```python
from build123d import *

# Parameters (mm, degrees)
F1_DEPTH = 15
F2_R     = 4
F3_DEPTH = 5


with BuildPart() as f1:
    # F0 (on Front) → F1 (new body, symmetric)
    with BuildSketch(Plane.XZ):
        with BuildLine():
            Line((0, 50), (-50, 50))
            Line((-50, 50), (-50, -50))
            Line((-50, -50), (0, -50))
            Line((0, -50), (0, -30))
            Line((0, -30), (-10, -30))
            ThreePointArc((-10, -30), (-18, -22.5), (-10, -15))
            Line((-10, -15), (0, -15))
            Line((0, -15), (0, 50))
        make_face()
    extrude(amount=F1_DEPTH, both=True)

    # F2 (on face) → F3 (cut)
    with BuildSketch(Plane.XZ.offset(15)):
        with Locations((-25, 25)):
            Circle(F2_R)
    extrude(amount=-F3_DEPTH, mode=Mode.SUBTRACT)


solid = f1.part
```
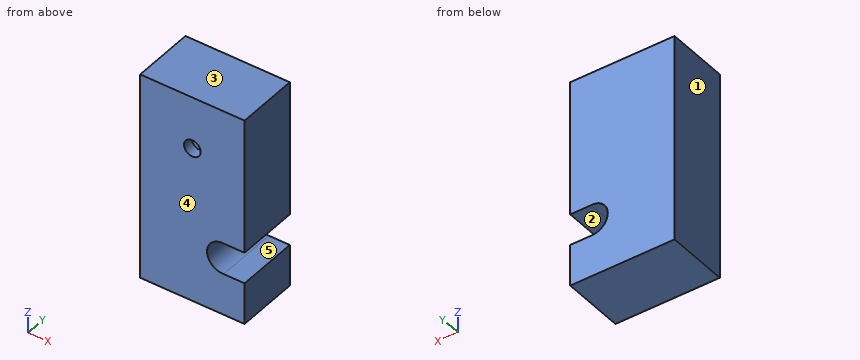
Source: CAD feature listing. Evaluate the final solid. Frame: model axes, mm. Face numbers are marked on the shaded views. A direction names the side the tool comes from. Give positions to 0.01 mm unless a question says otherwise; leave off trailing zeros. Loops run counter-clockwise (first coordinate to the right, second up) from the corner with the lowest first, then second, coordinate; pieces in that order, holes last. Notation, with made-up numbers: (24, 52.5) -> (38, 52.5) arc R12 cw to (38, 57.5) -> close; hole circle Ø9 at (24, 13.5). An arc over 180 degrees is marked (long way). Use a Markdown table: item, result. Add a question column.
(1) Section query C-C (y = -1.25). Output: boundary loops of the cut face in (x, z), then the cut area to 3 significant figures.
(2) Access query for the marked faces 4 and 5. Directions: +Z, -Z, +X, -X, +Y, -Y. A direction counts if a zero-diameter tool reaches every point of the face in a straight line with its end or side. Return the directions, or none.
(3) First-contact query: pin 1 Ø5 at (x, z) = (-25, 25) entering from -Y; pin 2 Ø9 at (x, z) = (-24, 25.5) entering from -Y. Flat tips, straight axial feed; report the tip coordinate or a pass-through.
(4) Pull-direction query (Z, two-part tool) for the marked faces 1, 2 and 3; classes: +Z half, -Z half, draft (parallel to the pull), parting line (faces both ways), or undercut.
(5) Section query B-B (y = -11.75). Output: boundary loops of the cut face in (x, z), then the cut area to 3 significant figures.
(6) Section query D-D (z = 25). Output: boundary loops of the cut face in (x, y), then the cut area to 3 significant figures.
(7) Ray query, line 1 (Z direction, x = -25, y = -12.35); line 2 (Z direction, x = -3, y = -9.5); line 3 (X direction, y = -1, z = -28.5). Return the intervals inside material, ascending.
(8) Section query A-A (x = -5.5). Output: boundary loops of the cut face in (y, z), then the cut area to 3 significant figures.
Checked values:
| question | item | result |
|---|---|---|
| 1 | outline | (-50, -50) -> (0, -50) -> (0, -30) -> (-10, -30) arc R7.52 cw (long way) to (-10, -15) -> (0, -15) -> (0, 50) -> (-50, 50) -> close |
| 1 | area | 4,750 mm^2 |
| 2 | face 4 | +Z, -Z, +X, -X, -Y |
| 2 | face 5 | +X, +Y, -Y |
| 3 | pin 1 | y = -10 |
| 3 | pin 2 | y = -15 |
| 4 | face 1 | draft |
| 4 | face 2 | undercut |
| 4 | face 3 | +Z half |
| 5 | outline | (-50, -50) -> (0, -50) -> (0, -30) -> (-10, -30) arc R7.52 cw (long way) to (-10, -15) -> (0, -15) -> (0, 50) -> (-50, 50) -> close; hole circle Ø8 at (-25, 25) |
| 5 | area | 4,700 mm^2 |
| 6 | outline | (-50, -15) -> (-29, -15) -> (-29, -10) -> (-21, -10) -> (-21, -15) -> (0, -15) -> (0, 15) -> (-50, 15) -> close |
| 6 | area | 1,460 mm^2 |
| 7 | line 1 | -50 to 21, 29 to 50 |
| 7 | line 2 | -50 to -30, -15 to 50 |
| 7 | line 3 | -50 to -15.01 |
| 8 | outline | (-15, -50) -> (15, -50) -> (15, -30) -> (-15, -30) -> close; (-15, -15) -> (15, -15) -> (15, 50) -> (-15, 50) -> close |
| 8 | area | 2,550 mm^2 |
